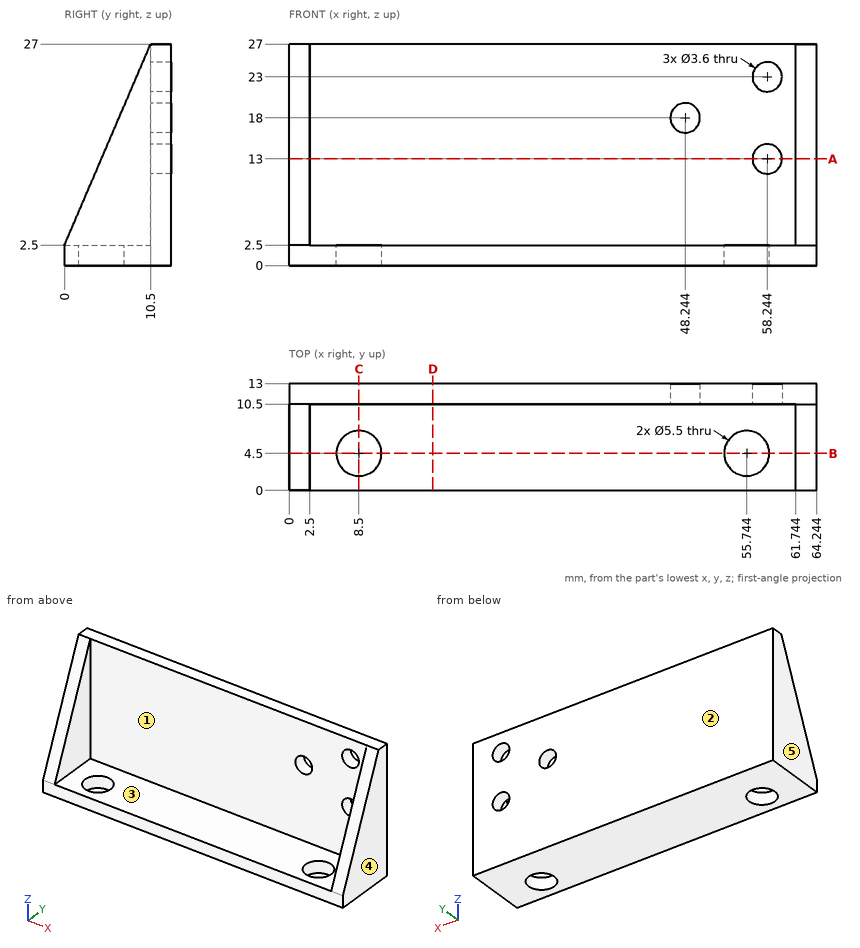
Answer from the drawing. Dimensions are ordinates in mm from the lowest x, y and z of the part. A direction names the side the tool comes from. Coordinates: 2 decimals unless noted, no trailing zeros. Loops run counter-clockwise (first coordinate to the right, second up) from the corner with the lowest first, then second, coordinate; pieces in that order, holes last. Notation, with made-up numbers: (73.25, -17) -> (98.25, -17) arc R23 cw to (98.25, 10) -> close; hole circle Ø6 at (29.5, 19). An arc over 180 degrees is marked (long way). Return JSON: item names as keys, results as strings.
Item 1: Find section C-C (x = 8.5). Determine the outline of the cut face in (y, z).
Answers:
{"outline": "(0, 0) -> (1.75, 0) -> (1.75, 2.5) -> (0, 2.5) -> close; (7.25, 0) -> (13, 0) -> (13, 27) -> (10.5, 27) -> (10.5, 2.5) -> (7.25, 2.5) -> close"}
Item 2: For a pull along X with two mould halves and no side action, classify the marked faces 3, 4 and 5 as +X half, -X half, draft (parallel to the pull), parting line (faces both ways), or undercut.
Answers:
{"face 3": "undercut", "face 4": "+X half", "face 5": "-X half"}
Item 3: Find section B-B (y = 4.5). Determine the outline of the cut face in (x, z).
Answers:
{"outline": "(0, 0) -> (5.75, 0) -> (5.75, 2.5) -> (2.5, 2.5) -> (2.5, 13) -> (0, 13) -> close; (11.25, 0) -> (52.99, 0) -> (52.99, 2.5) -> (11.25, 2.5) -> close; (58.49, 0) -> (64.24, 0) -> (64.24, 13) -> (61.74, 13) -> (61.74, 2.5) -> (58.49, 2.5) -> close"}
Item 4: Find section D-D (x = 17.5). Determine the outline of the cut face in (y, z).
Answers:
{"outline": "(0, 0) -> (13, 0) -> (13, 27) -> (10.5, 27) -> (10.5, 2.5) -> (0, 2.5) -> close"}
Item 5: Flat-ended cylindrical pins translate along their axes: P1, Ø4, axis at x = 15.5, z = 20.5, coming from the -Y side; P2, Ø3, axis at y = 6, z = 18, coming from the +X side. Find the tip coordinate at first contact, or state that the pin passes through.
Answers:
{"P1": "stops at y = 10.5", "P2": "stops at x = 64.24"}
Item 6: Find the intervals of material crossed by probe 1 along X at (y, z) = (4.5, 1.45); probe 2 along Y at (x, z) = (8.5, 1.3); probe 3 along X at (y, z) = (5, 11.5), in increasing order.
Answers:
{"probe 1": "x = 0 to 5.75, 11.25 to 52.99, 58.49 to 64.24", "probe 2": "y = 0 to 1.75, 7.25 to 13", "probe 3": "x = 0 to 2.5, 61.74 to 64.24"}
Item 7: For the marked faces 1 and 2, determine the directions among +Z, -Z, +X, -X, +Y, -Y from which every point of the face is accessible in a straight line to the end or side of a thin tool.
Answers:
{"face 1": "+Z, -Y", "face 2": "+Z, -Z, +X, -X, +Y"}
Item 8: Find section A-A (z = 13). Determine the outline of the cut face in (x, y).
Answers:
{"outline": "(0, 4.5) -> (2.5, 4.5) -> (2.5, 10.5) -> (56.44, 10.5) -> (56.44, 13) -> (0, 13) -> close; (60.04, 10.5) -> (61.74, 10.5) -> (61.74, 4.5) -> (64.24, 4.5) -> (64.24, 13) -> (60.04, 13) -> close"}
